Build history of the part. All positions in model axes, mm. Face numbers are marked on the shaded views. A direction names the side the tool comes from. Coordinates: 2 decimals unless noted, no trailing zeros. Loops run counter-clockwise (first coordinate to the right, second up) from the corner with the lowest first, then second, coordinate; pieces in that order, holes last.
Item 1: 3-axis set-ups, long thin cutter, end or side, ignore diameter. For the marked faces 1, 2, 3, 4 and 5: which of +Z, -Z, +X, -X, +Y, -Y reach the whole face in a straight line?
Item 2: Mould opens along Y. For the marked faces 6, 7 and 8 say: released by +Y, released by -Y, zero draft, split by the parting line, or undercut.
Item 3: Cut at C-C (x = 26.5). List the corners of the cut face in (y, z) (3 decimals).
Item 4: Drill centre lines: line 1 along Y through (x, z) = (-11.5, 35.25); line 2 along X through (y, z) = (-8, 7); line 3 along Z through (x, y) = (9, -9). Where is each one in solid material? Low to high.
Item 5: Flat gauge pins, fed straight in: pin 1 (4 mm diameter, centred on x = -8.5, y = 8.5, fed in from -Z); pin 2 (0.8 mm diameter, centred on x = 9.5, z = -3, fed in from -Y) (3 decimals); pin 3 (1.7 mm diameter, centred on y = 12.5, z = 32.5, fed in from -X). Where does each tip first touch, or does it go through?
Item 6: Cut at A-A (y = 0). List the corners of the cut face in (x, z), and give its area (3 significant figures).
Item 7: Cut at B-B (x = -5). List the corners of the cut face in (y, z), and give its area (3 significant figures).
Item 8: Cut at D-D (x = -35.5). List the corners of the cut face in (y, z).
from build123d import *

# Parameters (mm, degrees)
SKETCH_1_W                  = 65
SKETCH_1_H                  = 48
EXTRUDE_1_DEPTH             = 40
SKETCH_2_R                  = 3
CUT_EXTRUDE_1_DEPTH         = 6
HOLE_WIZARD_3_3_3_3_1_D     = 3.3
HOLE_WIZARD_3_3_3_3_1_DEPTH = 10
HOLE_WIZARD_3_3_3_3_1_TIP   = 0.991420021
SKETCH_5_R                  = 2.7
EXTRUDE_2_DEPTH             = 4
CUT_EXTRUDE_2_DEPTH         = 4
EXTRUDE_3_DEPTH             = 9
SKETCH_8_R                  = 3.3
EXTRUDE_4_DEPTH             = 4
CUT_EXTRUDE_3_DEPTH         = 4
SKETCH_11_R                 = 8
CUT_EXTRUDE_4_DEPTH         = 88.475710915
SKETCH_12_W                 = 1.91
SKETCH_12_H                 = 20.67
CUT_EXTRUDE_5_DEPTH         = 2.5
EXTRUDE_5_DEPTH             = 30


with BuildPart() as part:
    # 草图1 → 凸台-拉伸1 (new body)
    with BuildSketch(Plane.XY):
        Rectangle(SKETCH_1_W, SKETCH_1_H)
    extrude(amount=EXTRUDE_1_DEPTH)

    # 草图2 → 切除-拉伸1 (cut)
    with BuildSketch(Plane.XY.offset(40)):
        with Locations((22.5, 10)):
            Circle(SKETCH_2_R)
        with Locations((22.5, -10)):
            Circle(SKETCH_2_R)
        with Locations((7.5, 10)):
            Circle(SKETCH_2_R)
        with Locations((7.5, -10)):
            Circle(SKETCH_2_R)
    extrude(amount=-CUT_EXTRUDE_1_DEPTH, mode=Mode.SUBTRACT)

    # Ø3.3 (3.3) 直径孔1
    with Locations(Plane.XY.offset(40)):
        with Locations((13.5, -12.5), (-11.5, -12.5), (13.5, 12.5), (-11.5, 12.5)):
            Hole(HOLE_WIZARD_3_3_3_3_1_D / 2, depth=HOLE_WIZARD_3_3_3_3_1_DEPTH)
            with Locations((0, 0, -(HOLE_WIZARD_3_3_3_3_1_DEPTH + HOLE_WIZARD_3_3_3_3_1_TIP / 2))):  # 118° drill point
                Cone(0, HOLE_WIZARD_3_3_3_3_1_D / 2, HOLE_WIZARD_3_3_3_3_1_TIP, mode=Mode.SUBTRACT)

    # 草图5 → 凸台-拉伸2 (add)
    with BuildSketch(Plane.XY.offset(34)):
        with Locations((22.5, 10)):
            Circle(SKETCH_5_R)
        with Locations((7.5, 10)):
            Circle(SKETCH_5_R)
        with Locations((7.5, -10)):
            Circle(SKETCH_5_R)
        with Locations((22.5, -10)):
            Circle(SKETCH_5_R)
    extrude(amount=EXTRUDE_2_DEPTH)

    # 草图6 → 切除-拉伸2 (cut)
    with BuildSketch(Plane.XY.offset(38)):
        Polygon((24.341579714, -10.210975793), (23.603500253, -8.510633081), (21.761920539, -8.299657288), (20.658420286, -9.789024207), (21.396499747, -11.489366919), (23.238079461, -11.700342712), align=None)
        Polygon((5.794848806, -9.606351162), (6.30651451, -11.279879832), (8.011665703, -11.67352867), (9.205151194, -10.393648838), (8.69348549, -8.720120168), (6.988334297, -8.32647133), align=None)
        Polygon((21.45041022, 11.682057174), (20.518500867, 9.932057174), (21.568090646, 8.25), (23.54958978, 8.317942826), (24.481499133, 10.067942826), (23.431909354, 11.75), align=None)
        Polygon((5.873282152, 11.19880039), (5.648449484, 9.190621214), (7.275167332, 7.991820824), (9.126717848, 8.80119961), (9.351550516, 10.809378786), (7.724832668, 12.008179176), align=None)
    extrude(amount=-CUT_EXTRUDE_2_DEPTH, mode=Mode.SUBTRACT)

    # 草图7 → 凸台-拉伸3 (add)
    with BuildSketch(Plane.ZY.offset(32.5)):
        with BuildLine():
            Line((0, 13.266499161), (0, -13.266499161))
            ThreePointArc((0, -13.266499161), (20, -24), (40, -13.266499161))
            Line((40, -13.266499161), (40, 13.266499161))
            ThreePointArc((40, 13.266499161), (20, 24), (0, 13.266499161))
        make_face()
    extrude(amount=EXTRUDE_3_DEPTH)

    # 草图8 → 凸台-拉伸4 (add)
    with BuildSketch(Plane.ZY.offset(41.5)):
        with Locations(Location((20, 18, 0), (0, 0, 270))):
            Circle(SKETCH_8_R)
        with Locations(Location((32.727922061, 12.727922061, 0), (0, 0, 270))):
            Circle(SKETCH_8_R)
        with Locations(Location((7.272077939, 12.727922061, 0), (0, 0, 270))):
            Circle(SKETCH_8_R)
    extrude_4 = extrude(amount=EXTRUDE_4_DEPTH)

    # 草图9 → 切除-拉伸3 (cut)
    with BuildSketch(Plane.ZY.offset(45.5)):
        Polygon((5.811063185, 11.764627771), (7.375807889, 10.980999024), (8.836822642, 11.944293315), (8.733092692, 13.691216352), (7.168347989, 14.474845098), (5.707333235, 13.511550808), align=None)
        Polygon((31.486883058, 11.494097847), (33.175925673, 11.03623865), (34.416964676, 12.270062864), (33.968961065, 13.961746275), (32.27991845, 14.419605473), (31.038879446, 13.185781259), align=None)
        Polygon((18.478401074, 17.135571455), (19.987817617, 16.250042404), (21.509416543, 17.114470949), (21.521598926, 18.864428545), (20.012182383, 19.749957596), (18.490583457, 18.885529051), align=None)
    cut_extrude_3 = extrude(amount=-CUT_EXTRUDE_3_DEPTH, mode=Mode.SUBTRACT)

    # 镜向1: 凸台-拉伸4, 切除-拉伸3 across plane
    add(extrude_4.mirror(Plane.ZX))
    add(cut_extrude_3.mirror(Plane.ZX), mode=Mode.SUBTRACT)

    # 草图11 → 切除-拉伸4 (cut, through all)
    with BuildSketch(Plane.ZY.offset(41.5)):
        with Locations(Location((20, 0, 0), (0, 0, 270))):
            Circle(SKETCH_11_R)
    extrude(amount=-CUT_EXTRUDE_4_DEPTH, mode=Mode.SUBTRACT)

    # 草图12 → 切除-拉伸5 (cut)
    with BuildSketch(Plane(origin=(32.5, 0, 0), x_dir=(0, 0, -1), z_dir=(1, 0, 0))):
        with Locations((-0.955, 0)):
            Rectangle(SKETCH_12_W, SKETCH_12_H)
    extrude(amount=-CUT_EXTRUDE_5_DEPTH, mode=Mode.SUBTRACT)

    # 草图13 → 凸台-拉伸5 (add)
    with BuildSketch(Plane(origin=(30, 0, 0), x_dir=(0, 0, -1), z_dir=(1, 0, 0))):
        Polygon((-1.91, 10.335), (6.15, 10.335), (6.15, 5.995), (4.65, 5.995), (4.65, 4.495), (3.65, 4.495), (3.65, 5.995), (2.15, 5.995), (2.15, -5.995), (3.65, -5.995), (3.65, -4.495), (4.65, -4.495), (4.65, -5.995), (6.15, -5.995), (6.15, -10.335), (-1.91, -10.335), align=None)
    extrude(amount=-EXTRUDE_5_DEPTH)


solid = part.part
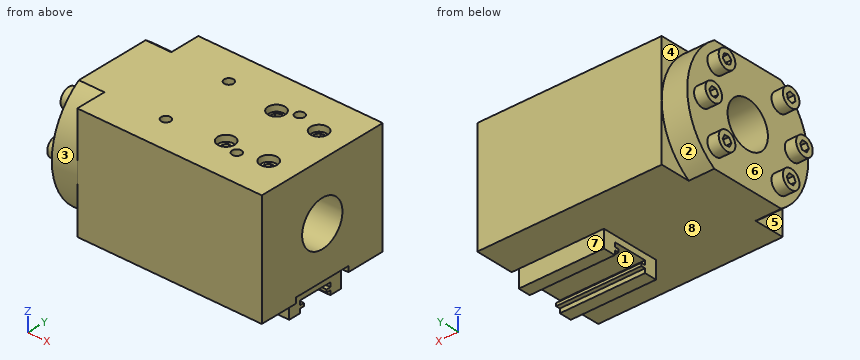
Filled sheet:
1. face 1: +X, -X
1. face 2: -X, +Y
1. face 3: -X, -Y
1. face 4: +Z, -X, +Y
1. face 5: -Z, -X, -Y
2. face 6: undercut
2. face 7: released by +Y
2. face 8: zero draft
3. outline: (-24, 0) - (-10.335, 0) - (-10.335, -6.15) - (-5.995, -6.15) - (-5.995, -4.65) - (-4.495, -4.65) - (-4.495, -3.65) - (-5.995, -3.65) - (-5.995, -2.15) - (5.995, -2.15) - (5.995, -3.65) - (4.495, -3.65) - (4.495, -4.65) - (5.995, -4.65) - (5.995, -6.15) - (10.335, -6.15) - (10.335, 0) - (24, 0) - (24, 40) - (-24, 40) - close; hole circle Ø16 at (0, 20)
4. line 1: y = -24 to -14.15, -10.85 to 10.85, 14.15 to 24
4. line 2: x = -41.5 to 32.5
4. line 3: z = -6.15 to 38
5. pin 1: stops at z = 0
5. pin 2: stops at y = -10.335
5. pin 3: stops at x = -41.5
6. outline: (-41.5, 0) - (0, 0) - (0, -2.15) - (30, -2.15) - (30, 1.91) - (32.5, 1.91) - (32.5, 12) - (-41.5, 12) - close; (-41.5, 28) - (32.5, 28) - (32.5, 40) - (-41.5, 40) - close
6. area: 1,840 mm2
7. outline: (-24, 0) - (24, 0) - (24, 40) - (-24, 40) - close; hole circle Ø16 at (0, 20)
7. area: 1,720 mm2
8. outline: (-13.27, 0) - (13.27, 0) arc R24 ccw to (13.27, 40) - (-13.27, 40) arc R24 ccw to start; hole circle Ø16 at (0, 20)
